Check sheet for the modelled part. Datum: model origin and axes. Units: mm. A direction names the side the tool comes from. Coordinates: 2 decimals unless noted, no trailing zeros. Write each loop counter-clockwise with the first axis right and the second up, starting at its lowest first coordinate (ties: lowest second). Pieces come first, ordered by that corner, then holes. Notation, with made-up numbers: (13.25, 41) -> (45.25, 41) arc R19 cw to (45.25, 78) -> close; hole circle Ø9 at (-32.5, 68). An arc over 180 degrees is marked (long way). One line per item, written item: value. Start each with the question number.
1) Sectioned sample at B-B on y = 29. Enter the section's corners in (x, z) (3 decimals).
2) Draft check along Z on faces 4 (the flat face through (20, 19, -3.175)), 5 (the cylindrical face through (18.91, 1.57, -3.18)), 6 (the flat face through (89, 19, -93.98)). Enter one of: +Z half, -Z half, draft (parallel to the pull), parting line (faces both ways), or undercut.
3) Gauge pin test, flat ends, axial feed: P1, Ø10, axis at x = -8.5, y = 12.5, coming from the +Z side; P2, Ø9.5, axis at x = 22, y = 14, coming from the -Z side (3 decimals); P3, Ø11.5, axis at y = 14.5, z = -41.5, coming from the -X side. Record the tip position at first contact, or that the pin passes through.
4) Sectioned sample at D-D on z = -6.35. Enter the section's corners in (x, y) (3 decimals), plus the area to 3 significant figures.
5) Set-up check for faces 1 (the flat face through (0, 19, -48)), 2 (the flat face through (3.175, 19, -50)), 3 (the flat face through (22, 38.1, -49)): record each of +Z, -Z, +X, -X, +Y, -Y from which the full face is reachable in a straight line by a thin tool's end or side.
6) Sectioned sample at A-A on x = 28.5. Enter the section's corners in (y, z) (3 decimals), plus the area to 3 significant figures.
7) Sectioned sample at C-C on z = -49. Enter the section's corners in (x, y) (3 decimals), plus the area to 3 significant figures.
8) Scan lines: line 1 along Y through (x, z) = (36.5, -66) (3 decimals); line 2 along Z through (x, y) = (19.05, 36.2) (3 decimals); line 3 along Z through (x, y) = (22, 9) (3 decimals). Record each from-to range of solid material in increasing order. Write a range as [from, to].
```python
from build123d import *

# Parameters (mm, degrees)
SKETCH1_R           = 3.175
BOSS_EXTRUDE1_DEPTH = 38.1
CUT_EXTRUDE1_START  = -34.925
CUT_EXTRUDE1_DEPTH  = 31.75


with BuildPart() as part:
    # Sketch1 → Boss-Extrude1 (new body)
    with BuildSketch(Plane(origin=(0, 0, 0), x_dir=(1, 0, 0), z_dir=(0, 1, 0))):
        Polygon((-12.7, 97.155), (-12.7, 93.98), (0, 93.98), (0, 0), (38.1, 0), (63.5, 93.98), (114.3, 93.98), (114.3, 97.155), align=None)
        with Locations(Location((19.05, 6.35, 0), (0, 0, 90))):
            Circle(SKETCH1_R, mode=Mode.SUBTRACT)
    extrude(amount=BOSS_EXTRUDE1_DEPTH)

    # Sketch2 → Cut-Extrude1 (cut)
    with BuildSketch(Plane.XZ.offset(CUT_EXTRUDE1_START)):
        Polygon((60.211083077, -97.155), (60.211083077, -93.98), (35.669191185, -3.175), (3.175, -3.175), (3.175, -93.98), (3.175, -97.155), align=None)
    extrude(amount=CUT_EXTRUDE1_DEPTH, mode=Mode.SUBTRACT)


solid = part.part
```
Answers:
1. outline: (-12.7, -97.155) -> (3.175, -97.155) -> (3.175, -3.175) -> (35.669, -3.175) -> (60.211, -93.98) -> (60.211, -97.155) -> (114.3, -97.155) -> (114.3, -93.98) -> (63.5, -93.98) -> (38.1, 0) -> (0, 0) -> (0, -93.98) -> (-12.7, -93.98) -> close
2. face 4: -Z half
2. face 5: undercut
2. face 6: +Z half
3. P1: stops at z = -93.98
3. P2: stops at z = -3.175
3. P3: stops at x = 0
4. outline: (0, 0) -> (15.875, 0) -> (15.875, 3.175) -> (3.175, 3.175) -> (3.175, 34.925) -> (15.875, 34.925) -> (15.875, 38.1) -> (0, 38.1) -> close; (22.225, 0) -> (39.816, 0) -> (39.816, 38.1) -> (22.225, 38.1) -> (22.225, 34.925) -> (36.527, 34.925) -> (36.527, 3.175) -> (22.225, 3.175) -> close
4. area: 418 mm2
5. face 1: +Z, -X, +Y, -Y
5. face 2: -Z
5. face 3: +Z, -Z, +X, -X, +Y
6. outline: (0, -97.155) -> (3.175, -97.155) -> (3.175, -3.175) -> (34.925, -3.175) -> (34.925, -97.155) -> (38.1, -97.155) -> (38.1, 0) -> (0, 0) -> close
6. area: 718 mm2
7. outline: (0, 0) -> (51.343, 0) -> (51.343, 38.1) -> (0, 38.1) -> close; hole (3.175, 3.175) -> (48.054, 3.175) -> (48.054, 34.925) -> (3.175, 34.925) -> close
7. area: 531 mm2
8. line 1: y = [0, 3.175], [34.925, 38.1]
8. line 2: z = [-97.155, -9.525], [-3.175, 0]
8. line 3: z = [-3.175, 0]
